Geometry: final body of the model. Coordinates: model frame, mm. A direction names the side the tool comes from. Give positions to 0.01 mm unless a question says otherwise; leave off trailing zeros. Loops run counter-clockwise (first coordinate to the right, second up) from the corner with the lowest first, then second, coordinate; pieces in that order, holes last. Notation, with made-up numbers: (6, 37) -> (28, 37) arc R20 ccw to (28, 75) -> close; hole circle Ø2 at (25.5, 23.25). An arc over 180 degrees is marked (long way). One line per item, written item: value. Start each with the question number.
from build123d import *

# Parameters (mm, degrees)
BASE_FLANGE1_DEPTH = 9.525
SKETCH6_R          = 1.905
CUT_EXTRUDE1_DEPTH = 26.173168455
SKETCH7_R          = 1.778
CUT_EXTRUDE2_DEPTH = 26.878337235
FILLET1_R          = 2.54


# Sheet-metal steps are written as plain solids
with BuildPart() as part:
    # Sketch2 → Base-Flange1 (new body)
    with BuildSketch(Plane.XY):
        with BuildLine():
            Line((0, 22.225), (0, 2.5748))
            ThreePointArc((0, 2.5748), (0.75414146, 0.75414146), (2.5748, 0))
            Line((2.5748, 0), (10.795, 0))
            Line((10.795, 0), (10.795, 1.5748))
            Line((10.795, 1.5748), (2.5748, 1.5748))
            ThreePointArc((2.5748, 1.5748), (1.867693219, 1.867693219), (1.5748, 2.5748))
            Line((1.5748, 2.5748), (1.5748, 22.225))
            Line((1.5748, 22.225), (0, 22.225))
        make_face()
    extrude(amount=BASE_FLANGE1_DEPTH)

    # Sketch6 → Cut-Extrude1 (cut, through all)
    with BuildSketch(Plane(origin=(0, 1.5748, 0), x_dir=(1, 0, 0), z_dir=(0, 1, 0))):
        with Locations(Location((7.0612, -4.7625, 0), (0, 0, 270))):
            Circle(SKETCH6_R)
    extrude(amount=-CUT_EXTRUDE1_DEPTH, mode=Mode.SUBTRACT)

    # Sketch7 → Cut-Extrude2 (cut, through all)
    with BuildSketch(Plane(origin=(1.5748, 0, 0), x_dir=(0, 0, -1), z_dir=(1, 0, 0))):
        with Locations((-4.7625, 19.05)):
            Circle(SKETCH7_R)
    extrude(amount=-CUT_EXTRUDE2_DEPTH, mode=Mode.SUBTRACT)

    # Fillet1
    fillet1_edges = [part.edges().sort_by_distance(p)[0] for p in [
        (10.795, 0.7874, 9.525),
        (0.7874, 22.225, 9.525),
        (10.795, 0.7874, 0),
        (0.7874, 22.225, 0),
    ]]
    fillet(fillet1_edges, radius=FILLET1_R)


solid = part.part
Item 1: Pin query (flat end, axial travel): pin 1 (1.5 mm diameter, centred on x = 4, y = 10, fed in from -Z); pin 2 (3 mm diameter, centred on y = 11, z = 2.5, fed in from +X). Return the tip coordinate at first contact, or that it passes through.
Item 2: Ray query, line 1 along Y through (x, z) = (5.5, 1); line 2 along Z through (x, y) = (0.5, 17.5) (3 decimals). Return the intervals inside material, ascending. Write a range as [from, to].
Item 3: Access query for faces 1 (the face through (0.798, 20.813, 4.994)), 2 (the face through (5, 1.575, 5)). Directions: +Z, -Z, +X, -X, +Y, -Y. A direction counts if a zero-diameter tool reaches every point of the face in a straight line with its end or side. Return the directions, or none.
Item 4: Section A-A, the plane y = 19.05. Output: boundary loops of the cut face in (x, z) (1 decimal).
Item 5: Section D-D, the plane y = 11.5. Output: boundary loops of the cut face in (x, z) (3 decimals).
Item 6: Section C-C, the plane z = 8.5. Output: boundary loops of the cut face in (x, y).
Item 7: Mould query, pull axis Z, two halves, no side actions, for faces 3 (the face through (5.2, 0.8, 4.35)), 4 (the face through (0.776, 21.501, 0.764)), 5 (the face through (10.795, 1, 5)). Classes: pulls with the +Z half, pulls with the -Z half, needs draft (parallel to the pull), parting line crosses it, or undercut.
Item 8: Section B-B, the plane x = 6. Output: boundary loops of the cut face in (y, z) (3 decimals).
Geometry check:
1. pin 1: passes through
1. pin 2: stops at x = 1.57
2. line 1: y = [0, 1.57]
2. line 2: z = [0, 3.891], [5.634, 9.525]
3. face 1: +X, -X
3. face 2: +Z, -Z, +X, +Y
4. outline: (0, 0) -> (1.6, 0) -> (1.6, 3) -> (0, 3) -> close; (0, 6.5) -> (1.6, 6.5) -> (1.6, 9.5) -> (0, 9.5) -> close
5. outline: (0, 0) -> (1.575, 0) -> (1.575, 9.525) -> (0, 9.525) -> close
6. outline: (0, 2.57) arc R2.57 ccw to (2.57, 0) -> (10.29, 0) -> (10.29, 1.57) -> (2.57, 1.57) arc R1 cw to (1.57, 2.57) -> (1.57, 21.72) -> (0, 21.72) -> close
7. face 3: undercut
7. face 4: pulls with the -Z half
7. face 5: needs draft
8. outline: (0, 0) -> (1.575, 0) -> (1.575, 3.18) -> (0, 3.18) -> close; (0, 6.345) -> (1.575, 6.345) -> (1.575, 9.525) -> (0, 9.525) -> close
